For this review, take the finished solid that the model builds, in its own axes (mm). Face numbers are marked on the shaded views. A direction names the side the tool comes from. Give positions to 0.01 mm unless a question says otherwise; leave off trailing zeros. Loops run counter-clockwise (first coordinate to the right, second up) from the corner with the lowest first, then second, coordinate; pieces in that order, holes last. Notation, with made-up numbers: (-18.75, -9) - (27.25, -9) arc R25 ccw to (27.25, 30) - close; hole circle Ø6 at (10.5, 6.5). An arc over 180 degrees is marked (long way). Use CSV: the item, a comma, the result in double quotes. Start each with the question number.
1. Wall thickness on line 1 (Y direction, x = -6.55, z = 11); line 2 (Z direction, x = -18.5, y = 48); line 3 (Y direction, x = -20.5, z = -10): over which ranges is each line inside the solid? List them lowest first.
2. Mouldability with a two-part tool opening along Z and no side actions: class the marked faces 4, 5 and 6 as pulls with the +Z half, pulls with the -Z half, needs draft (parallel to the pull), parting line crosses it, or undercut.
3. Take a section at B-B on y = 64. Give the boundary of the cut face in (x, z).
4. Take a section at A-A on z = 5. Give the boundary of the cut face in (x, y) (3 decimals), plus the area to 3 significant figures.
5. For the marked faces 1, 2 and 3, list the 3-axis set-ups (+Z, -Z, +X, -X, +Y, -Y) from which the entire face can be reached by the end or side of a thin tool; tool diameter is ignored.
6. For pin 1 (1.6 mm diameter, centred on x = 6.5, z = 5.5, fed in from -Y); pin 2 (9.5 mm diameter, centred on y = 11.5, z = 8, fed in from +X); pin 3 (10 mm diameter, centred on x = 7, z = 10, fed in from +Y), all flat-tipped, find the tip position at first contact; note any pin that passes through.
7. Take a section at C-C on x = 17. Give the boundary of the cut face in (y, z).
8. Take a section at D-D on z = -9. Give the boundary of the cut face in (x, y), plus the area to 3 significant figures.
```python
from build123d import *

# Parameters (mm, degrees)
BOSS_EXTRUDE1_DEPTH = 25
CHAMFER1_SIZE       = 7.62
CHAMFER1_SIZE2      = 12.7
CHAMFER2_SIZE       = 12.7
CHAMFER2_SIZE2      = 7.62
SKETCH2_W           = 12.5
SKETCH2_H           = 49.53232107
SKETCH2_H_2         = 15.55880868
CUT_EXTRUDE1_DEPTH  = 93.888113341
CHAMFER3_SIZE       = 10
CUT_EXTRUDE2_DEPTH  = 10
CHAMFER4_SIZE       = 4
SKETCH4_W           = 3.25
SKETCH4_H           = 12
SKETCH4_W_2         = 1.625
BOSS_EXTRUDE2_DEPTH = 17
FILLET1_R           = 6
SKETCH5_R           = 2
CUT_EXTRUDE3_DEPTH  = 96.527229626


# Some blends are built 0.0001 mm under size
with BuildPart() as part:
    # Sketch1 → Boss-Extrude1 (new, symmetric)
    with BuildSketch(Plane(origin=(0, 0, 0), x_dir=(0, 0, -1), z_dir=(1, 0, 0))):
        Polygon((2.54, 77.46), (38.54, 77.46), (38.54, 74), (40.04, 74), (40.04, 80), (0, 80), (0, 0), (24.04, 0), (24.04, 5.04), (22.54, 5.04), (22.54, 2.54), (2.54, 2.54), align=None)
    extrude(amount=BOSS_EXTRUDE1_DEPTH, both=True)

    # Chamfer1
    chamfer1_edges = [part.edges().sort_by_distance(p)[0] for p in [
        (0, 77.46, -2.54),
    ]]
    chamfer1_side = [part.faces().sort_by_distance(p)[0] for p in [
        (0, 40, -2.54),
    ]]
    chamfer(chamfer1_edges, length=CHAMFER1_SIZE, length2=CHAMFER1_SIZE2, reference=chamfer1_side[0])

    # Chamfer2
    chamfer2_edges = [part.edges().sort_by_distance(p)[0] for p in [
        (0, 80, 0),
    ]]
    chamfer2_side = [part.faces().sort_by_distance(p)[0] for p in [
        (0, 80, -20.02),
    ]]
    chamfer(chamfer2_edges, length=CHAMFER2_SIZE, length2=CHAMFER2_SIZE2, reference=chamfer2_side[0])

    # Sketch2 → Cut-Extrude1 (cut, through all)
    with BuildSketch(Plane.XY):
        Polygon((25, 0), (3.890569181, 0), (3.890569181, -6.225652432), (33.580070914, -6.225652432), (33.580070914, 22.733692281), (25, 22.733692281), align=None)
        Polygon((25, 22.733692281), (3.890569181, 0), (25, 0), align=None)
        with Locations((-6.25, 47.613839465)):
            Rectangle(SKETCH2_W, SKETCH2_H)
        with Locations((6.25, 47.613839465)):
            Rectangle(SKETCH2_W, SKETCH2_H)
        with Locations((6.25, 80.15940434)):
            Rectangle(SKETCH2_W, SKETCH2_H_2)
        with Locations((-6.25, 80.15940434)):
            Rectangle(SKETCH2_W, SKETCH2_H_2)
        Polygon((-33.580070914, 22.733692281), (-25, 22.733692281), (-3.890569181, 0), (-3.890569181, -6.225652432), (-33.580070914, -6.225652432), align=None)
    extrude(amount=-CUT_EXTRUDE1_DEPTH, mode=Mode.SUBTRACT)

    # Chamfer3
    chamfer3_edges = [part.edges().sort_by_distance(p)[0] for p in [
        (12.5, 22.84767893, -1.27),
        (-12.5, 22.84767893, -1.27),
    ]]
    chamfer(chamfer3_edges, length=CHAMFER3_SIZE)

    # Sketch3 → Cut-Extrude2 (cut)
    with BuildSketch(Plane.XZ):
        Polygon((6.24909298, -2.54), (2.09252957, -27.477990004), (-2.09252957, -27.477990004), (-6.24909298, -2.54), (-9.067628135, -2.54), (-9.067628135, -35.311562239), (9.067628135, -35.311562239), (9.067628135, -2.54), align=None)
    extrude(amount=-CUT_EXTRUDE2_DEPTH, mode=Mode.SUBTRACT)

    # Chamfer4
    # the kernel refuses this chamfer: 4 mm, written as the material it adds along each edge
    with BuildSketch(Plane(origin=(16.535824932, 2.54, -2.54), x_dir=(0, 0.9996219169112968, 0.027495876610586494), z_dir=(-1, 0, 0))) as chamfer4_piece_1_section:
        Polygon((CHAMFER4_SIZE * 0.999621916911, CHAMFER4_SIZE * 0.0274958766106), (-CHAMFER4_SIZE * 0.0274958766106, CHAMFER4_SIZE * 0.999621916911), (0, 0), align=None)
    chamfer4_piece_1 = extrude(amount=33.071649864, mode=Mode.PRIVATE)
    chamfer4_piece_1 = split(chamfer4_piece_1, bisect_by=Plane(origin=(-5.870802052, 3.874203196, -4.809619019), z_dir=(0.9863924373611449, 0, 0.16440790588271567)), keep=Keep.TOP, mode=Mode.PRIVATE)
    chamfer4_piece_1 = split(chamfer4_piece_1, bisect_by=Plane(origin=(5.870802052, 3.874203196, -4.809619019), z_dir=(-0.9863924373611449, 0, 0.16440790588271567)), keep=Keep.TOP, mode=Mode.PRIVATE)
    add(chamfer4_piece_1)
    # the kernel refuses this chamfer: 4 mm, written as the material it takes off along each edge
    with BuildSketch(Plane(origin=(-14.177301133, 0, 0), x_dir=(0, 0.9996219169112968, 0.027495876610586372), z_dir=(1, 0, 0))) as chamfer4_2_piece_1:
        Polygon((CHAMFER4_SIZE * 0.999621916911, -CHAMFER4_SIZE * 0.0274958766106), (-CHAMFER4_SIZE * 0.0274958766106, -CHAMFER4_SIZE * 0.999621916911), (0, 0), align=None)
    extrude(amount=28.354602266, mode=Mode.SUBTRACT)

    # Sketch4 → Boss-Extrude2 (add)
    with BuildSketch(Plane.XY):
        with Locations((-6.875, 11.84767893)):
            Rectangle(SKETCH4_W, SKETCH4_H)
        with Locations((0.8125, 11.84767893)):
            Rectangle(SKETCH4_W_2, SKETCH4_H)
        with Locations((-0.8125, 11.84767893)):
            Rectangle(SKETCH4_W_2, SKETCH4_H)
        with Locations((6.875, 11.84767893)):
            Rectangle(SKETCH4_W, SKETCH4_H)
    extrude(amount=BOSS_EXTRUDE2_DEPTH)

    # Fillet1
    fillet1_edges = [part.edges().sort_by_distance(p)[0] for p in [
        (-6.875, 5.84767893, 17),
        (0, 5.84767893, 17),
        (6.875, 5.84767893, 17),
        (6.875, 17.84767893, 17),
        (0, 17.84767893, 17),
        (-6.875, 17.84767893, 17),
    ]]
    fillet(fillet1_edges, radius=FILLET1_R - 0.0001)  # a hair under: the kernel refuses the full size

    # Sketch5 → Cut-Extrude3 (cut, through all)
    with BuildSketch(Plane(origin=(8.5, 0, 0), x_dir=(0, 0, -1), z_dir=(1, 0, 0))):
        with Locations((-11, 11.84767893)):
            Circle(SKETCH5_R)
    extrude(amount=-CUT_EXTRUDE3_DEPTH, mode=Mode.SUBTRACT)


solid = part.part
```
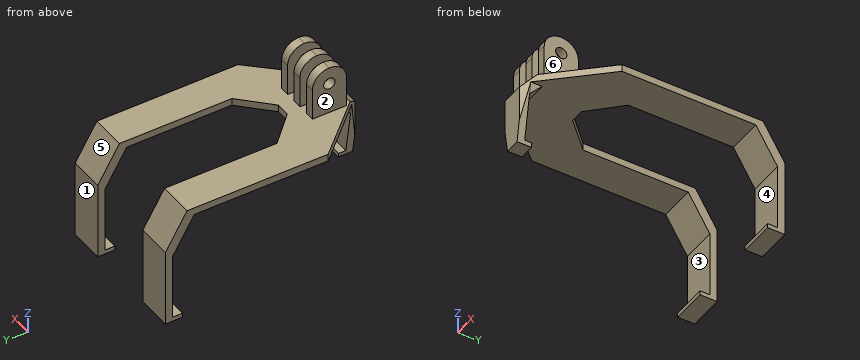
Check result:
1,line 1,"y = 5.85 to 9.85, 13.85 to 17.85"
1,line 2,"z = -2.54 to 0"
1,line 3,"y = 74.32 to 78.38"
2,face 4,"undercut"
2,face 5,"pulls with the +Z half"
2,face 6,"needs draft"
3,outline,"(-25, -2.54) - (-12.5, -2.54) - (-12.5, 0) - (-25, 0) - close; (12.5, -2.54) - (25, -2.54) - (25, 0) - (12.5, 0) - close"
4,outline,"(-8.5, 5.848) - (-5.25, 5.848) - (-5.25, 17.848) - (-8.5, 17.848) - close; (-1.625, 5.848) - (1.625, 5.848) - (1.625, 17.848) - (-1.625, 17.848) - close; (5.25, 5.848) - (8.5, 5.848) - (8.5, 17.848) - (5.25, 17.848) - close"
4,area,"117 mm²"
5,face 1,"+Z, -Z, +X, -X, +Y"
5,face 2,"+Z, -X, +Y, -Y"
5,face 3,"+X, -X, -Y"
6,pin 1,"stops at y = 5.85"
6,pin 2,"stops at x = 8.5"
6,pin 3,"stops at y = 17.85"
7,outline,"(14.12, -2.54) - (69.84, -2.54) - (77.46, -15.24) - (77.46, -38.54) - (74, -38.54) - (74, -40.04) - (80, -40.04) - (80, -12.7) - (72.38, 0) - (14.12, 0) - close"
8,outline,"(-25, 73.72) - (-12.5, 73.72) - (-12.5, 77.78) - (-25, 77.78) - close; (-5.17, 1.38) - (-3.89, 0) - (3.89, 0) - (5.17, 1.38) - (5.17, 2.54) - (-5.17, 2.54) - close; (12.5, 73.72) - (25, 73.72) - (25, 77.78) - (12.5, 77.78) - close"
8,area,"126 mm²"
